from build123d import *

# Parameters (mm, degrees)
F0_R     = 46.5439630146
F1_DEPTH = 25.4
F2_T     = -2.54
F3_R     = 26.6785648963
F4_DEPTH = 38.1
F5_T     = 2.54


# Not quite as in the source:
# - a fillet or chamfer that OpenCascade refuses, or shapes differently, is made with other operations: its cross-section is extruded or revolved along the edge and cut away or added
# - a shell that OpenCascade refuses in one call is made with other operations: the cavity is built on its own and cut out


with BuildPart() as f1:
    # F0 (on Right) → F1 (new body)
    with BuildSketch(Plane.YZ):
        Circle(F0_R)
    extrude(amount=F1_DEPTH)

    # F2
    f2_openings = [f1.faces().sort_by_distance(p)[0] for p in [
        (0, 0, 0),
    ]]
    offset(amount=F2_T, openings=f2_openings)

    # F3 (on face) → F4 (join)
    with BuildSketch(Plane.YZ.offset(25.4)):
        Circle(F3_R)
    extrude(amount=F4_DEPTH)

    # F5: shell of thickness 2.54, made by hand


with BuildPart() as f5_core1:
    # F5_t2: copy of F1
    add(f1.part)

    # the walls: a layer under each face that stays
    f5_faces = [f5_core1.faces().sort_by_distance(p)[0] for p in [
        (12.7, -46.5439630146, 0),
        (0, -43.441032147, -12.4117234706),
        (11.43, -44.0039630146, 0),
        (44.45, -26.6785648963, 0),
        (22.86, 0, 0),
        (63.5, 0, 0),
    ]]
    thicken(f5_faces, amount=-F5_T, mode=Mode.SUBTRACT)

    # F5_s3 → F5_t4 (revolve, cut)
    with BuildSketch(Plane.XY):
        Polygon((22.8346, 43.9785630146), (22.86, 46.5439630146), (25.4, 46.5439630146), (25.4, 44.0039630146), align=None)
    revolve(axis=Axis((22.86, 0, 0), (-1, 0, 0)), mode=Mode.SUBTRACT)


with BuildPart() as f1_1:
    add(f1.part)

    # what is left inside the walls is the cavity
    f5_cavity = [f5_core1.part.solids().sort_by_distance(p)[0] for p in [
        (49.106667, -24.113165, 0),
    ]]
    add(f5_cavity, mode=Mode.SUBTRACT)

    # F6: fillet of radius 5.08 on 3 edges, made by hand

    # F6_s1 → F6_t2 (revolve, cut)
    with BuildSketch(Plane.XY):
        with BuildLine():
            ThreePointArc((4.3999665546, 46.5443630146), (1.8595251638, 45.8637284922), (-0.0003463882, 44.0041630527))
            Line((-0.0003463882, 44.0041630527), (-0.4403776825, 44.258279625))
            ThreePointArc((-0.4403776825, 44.258279625), (-0.5081365685, 45.2740630337), (-0.5081365685, 46.5439630146))
            Line((-0.5081365685, 46.5439630146), (0, 47.0520995832))
            ThreePointArc((0, 47.0520995832), (2.1999832773, 47.0520995832), (4.3999665546, 47.0524995832))
            Line((4.3999665546, 47.0524995832), (4.3999665546, 46.5443630146))
        make_face()
    revolve(axis=Axis((0, 0, 0), (1, 0, 0)), mode=Mode.SUBTRACT)

    # F6_s3 → F6_t4 (revolve, cut)
    with BuildSketch(Plane.XY):
        with BuildLine():
            ThreePointArc((20.3190343146, 46.5443630146), (23.9121024484, 45.0560654631), (25.4004, 41.4629973292))
            Line((25.4004, 41.4629973292), (25.9085365685, 41.4629973292))
            ThreePointArc((25.9085365685, 41.4629973292), (25.9081365685, 44.0034801719), (25.9081365685, 46.5439630146))
            Line((25.9081365685, 46.5439630146), (25.4, 47.0520995832))
            ThreePointArc((25.4, 47.0520995832), (22.8595171573, 47.0520995832), (20.3190343146, 47.0524995832))
            Line((20.3190343146, 47.0524995832), (20.3190343146, 46.5443630146))
        make_face()
    revolve(axis=Axis((25.4, 0, 0), (1, 0, 0)), mode=Mode.SUBTRACT)

    # F6_s5 → F6_t6 (revolve, cut)
    with BuildSketch(Plane.XY):
        with BuildLine():
            ThreePointArc((58.4190343146, 26.6789648963), (62.0121024484, 25.1906673448), (63.5004, 21.5975992109))
            Line((63.5004, 21.5975992109), (64.0085365685, 21.5975992109))
            ThreePointArc((64.0085365685, 21.5975992109), (64.0081365685, 24.1380820536), (64.0081365685, 26.6785648963))
            Line((64.0081365685, 26.6785648963), (63.5, 27.1867014649))
            ThreePointArc((63.5, 27.1867014649), (60.9595171573, 27.1867014649), (58.4190343146, 27.1871014649))
            Line((58.4190343146, 27.1871014649), (58.4190343146, 26.6789648963))
        make_face()
    revolve(axis=Axis((63.5, 0, 0), (1, 0, 0)), mode=Mode.SUBTRACT)


solid = f1_1.part
Design review of the part built by this model. Coordinates are the model's own, in mm. A direction names the side the tool comes from. Round coordinates to 2 decimals unless told otherwise and drop trailing zeros. Order: outer loops, then holes, each group sorted by start corner. A loop starts at its lowest first (then second) coordinate and runs counter-clockwise, first axis right, second up.
1) Consider section D-D (x = 15). State the section outline as (y, z) points.
The answers:
outline: circle Ø93.09 at (0, 0); hole circle Ø88.01 at (0, 0)
2) Consider section C-C (x = 53). State the section outline as (y, z) points.
The answers:
outline: circle Ø53.36 at (0, 0); hole circle Ø48.28 at (0, 0)
3) For L1, parallel to Z at x = 38, y = 0; L2, parallel to Z at x = 9.25, y = 0, list the stretches that pass through material, from the lowest coordinate up.
The answers:
L1: z = -26.68 to -24.14, 24.14 to 26.68
L2: z = -46.54 to -44, 44 to 46.54
4) Machinability: for faces 4 (the flat face through (22.86, -1, 1)), 5 (the cylindrical face through (41.71, 25.447, 8.014)), 6 (the cylindrical face through (42.931, -19.156, -14.688)), which of the approach directions +Z, -Z, +X, -X, +Y, -Y give a long, thin tool a straight path to every point of the face, cutting with its end or side? Answer none if there is none.
The answers:
face 4: -X
face 5: +X
face 6: none
5) Draft analysis for pull direction Z (two halves, no side actions). For faces 1 (the flat face through (60.96, 0, 0)), 2 (the flat face through (25.4, -1, -27)), 3 (the cylindrical face through (12.247, -36.936, -28.321)), state which applies: released by +Z, released by -Z, zero draft, split by the parting line, or undercut.
The answers:
face 1: undercut
face 2: zero draft
face 3: split by the parting line
6) Clearance check with flat-ended pins moving along their axes: pin 1 Ø14.5 at (y, z) = (3.5, -8.5) entering from -X; pin 2 Ø1 at (x, z) = (19.5, -25) entering from -Y; pin 3 Ø12 at (x, z) = (45, 21.5) entering from -Y. State where each tip first meets the part, or that it passes through.
The answers:
pin 1: stops at x = 22.86
pin 2: stops at y = -39.57
pin 3: stops at y = -21.71
